from build123d import *

# Parameters (mm, degrees)
BOSS_EXTRU_1_DEPTH = 12.4
BOSS_EXTRU_2_DEPTH = 5.6
ESQUISSE3_R        = 2.35
BOSS_EXTRU_3_DEPTH = 5.2
ESQUISSE4_R        = 3.5
BOSS_EXTRU_4_DEPTH = 3.7


with BuildPart() as part:
    # Esquisse1 → Boss.-Extru.1 (new body)
    with BuildSketch(Plane.XY):
        Polygon((-11.4, 10), (-16.3, 10), (-16.3, 7.1), (-11.4, 7.1), (-11.4, -11.4), (11.4, -11.4), (11.4, 7.1), (16.3, 7.1), (16.3, 10), (11.4, 10), (11.4, 11.4), (-11.4, 11.4), align=None)
    extrude(amount=BOSS_EXTRU_1_DEPTH)

    # Esquisse2 → Boss.-Extru.2 (add)
    with BuildSketch(Plane(origin=(0, 11.4, 0), x_dir=(1, 0, 0), z_dir=(0, 1, 0))):
        with BuildLine():
            Line((-1.35, -3.75), (-0.495392875, -3.75))
            ThreePointArc((-0.495392875, -3.75), (11.4, -6.2), (-0.495392875, -8.65))
            Line((-0.495392875, -8.65), (-1.35, -8.65))
            ThreePointArc((-1.35, -8.65), (-3.8, -6.2), (-1.35, -3.75))
        make_face()
    extrude(amount=BOSS_EXTRU_2_DEPTH)

    # Esquisse3 → Boss.-Extru.3 (add)
    with BuildSketch(Plane(origin=(0, 17, 0), x_dir=(1, 0, 0), z_dir=(0, 1, 0))):
        with Locations(Location((5.2, -6.2, 0), (0, 0, 270))):
            Circle(ESQUISSE3_R)
    extrude(amount=BOSS_EXTRU_3_DEPTH)

    # Esquisse4 → Boss.-Extru.4 (add)
    with BuildSketch(Plane(origin=(0, 22.2, 0), x_dir=(1, 0, 0), z_dir=(0, 1, 0))):
        with Locations(Location((5.2, -6.2, 0), (0, 0, 270))):
            Circle(ESQUISSE4_R)
    extrude(amount=-BOSS_EXTRU_4_DEPTH)


solid = part.part
The model under review builds one solid part; all positions refer to its coordinate system, in mm. A direction names the side the tool comes from. Round coordinates to 2 decimals unless told otherwise and drop trailing zeros. Order: outer loops, then holes, each group sorted by start corner. A loop starts at its lowest first (then second) coordinate and runs counter-clockwise, first axis right, second up. Notation, with made-up numbers: (48.25, -25.75) -> (93.25, -25.75) arc R27 cw to (93.25, -4.75) -> close; hole circle Ø3 at (73.5, 16). An arc over 180 degrees is marked (long way). Use CSV: the item, a comma, the result in double quotes. Start each with the question number.
(1) Mouldability with a two-part tool opening along Y and no side actions: class faces 1 (the face through (14, 7.1, 6)), 2 (the face through (11.4, -2, 6)), 3 (the face through (-7, 11.4, 6)), 4 (the face through (3, 18.5, 5)) as pulls with the +Y half, pulls with the -Y half, needs draft (parallel to the pull), parting line crosses it, or undercut.
(2) Wall thickness on probe 1 along Y at (x, z) = (8, 8); probe 2 along X at (y, z) = (3.5, 11.75): over which ranges is each line inside the solid? List them lowest first. Write a range as from..to.
(3) Insertion check: pin 1 (1.9 mm diameter, centred on x = 8, z = 2, fed in from +Y); pin 2 (2.5 mm diameter, centred on x = 14.5, z = 9.5, fed in from -Y); pin 3 (1.5 mm diameter, centred on y = 12.5, z = 2, fed in from -X). Each pin has a flat end and moves straight along its axis. Give the tip position at first contact, or say it passes through.
(4) Tool access review of faces 5 (the face through (10, 11.4, 1)), 6 (the face through (-11.4, 11, 6)), 7 (the face through (2, 17, 6)): name each direction out of +Z, -Z, +X, -X, +Y, -Y from which nothing blocks a thin tool from reaching the whole face with its end or side.
(5) Consider section C-C on y = 13.5. Write out the cut boundary in (x, z).
(6) Consider section B-B on y = 18. Write out the cut boundary in (x, z), and give its area (3 significant figures).
(7) Consider section A-A on x = -8.5. Write out the cut boundary in (y, z).
Responses:
1,face 1,"pulls with the -Y half"
1,face 2,"needs draft"
1,face 3,"pulls with the +Y half"
1,face 4,"undercut"
2,probe 1,"-11.4..17, 18.5..22.2"
2,probe 2,"-11.4..11.4"
3,pin 1,"y = 17"
3,pin 2,"y = 7.1"
3,pin 3,"x = 0.05"
4,face 5,"-Z, +X, +Y"
4,face 6,"+Z, -Z, -X, +Y"
4,face 7,"none"
5,outline,"(-1.35, 3.75) -> (-0.5, 3.75) arc R6.2 ccw (long way) to (-0.5, 8.65) -> (-1.35, 8.65) arc R2.45 ccw to start"
6,outline,"circle Ø4.7 at (5.2, 6.2)"
6,area,"17.3 mm²"
7,outline,"(-11.4, 0) -> (11.4, 0) -> (11.4, 12.4) -> (-11.4, 12.4) -> close"
